```python
from build123d import *

# Parameters (mm, degrees)
F0_R     = 5.25
F0_R_2   = 4.25
F1_DEPTH = 6


with BuildPart() as f1:
    # F0 (on Front) → F1 (new body)
    with BuildSketch(Plane.XZ):
        with BuildLine():
            Line((-25, 25), (-25, 0))
            ThreePointArc((-25, 0), (0, -25), (25, 0))
            Line((25, 0), (25, 110))
            ThreePointArc((25, 110), (16.706063, 126.216291), (-1.296809, 128.982892))
            Line((-1.296809, 128.982892), (-167.871012, 73.728615))
            ThreePointArc((-167.871012, 73.728615), (-184.680107, 46.013484), (-160, 25))
            Line((-160, 25), (-25, 25))
        make_face()
        with Locations((-160, 50)):
            Circle(F0_R, mode=Mode.SUBTRACT)
        Circle(F0_R_2, mode=Mode.SUBTRACT)
    extrude(amount=F1_DEPTH)


solid = f1.part
```
Work out the finished part from the listing and answer in its coordinate system (mm). A direction names the side the tool comes from. Give positions to 0.01 mm unless a question says otherwise; leave off trailing zeros. Loops run counter-clockwise (first coordinate to the right, second up) from the corner with the lowest first, then second, coordinate; pieces in that order, holes last. Notation, with made-up numbers: (55, 86.5) -> (69, 86.5) arc R21 ccw to (69, 113.5) -> close; hole circle Ø2 at (69.25, 56.25). An arc over 180 degrees is marked (long way). Use CSV: the item, a comma, the result in double quotes.
1. The part is cut by section D-D (z = 86). Write down the section's boundary in (x, y).
Found:
outline,"(-130.88, -6) -> (25, -6) -> (25, 0) -> (-130.88, 0) -> close"
2. Flat-ended cylindrical pins translate along their axes: pin 1 Ø1.5 at (x, y) = (-29, -0.5) entering from +Z; pin 2 Ø9.5 at (x, z) = (-160, 50) entering from +Y. Find the tip coordinate at first contact, or state that the pin passes through.
Found:
pin 1,"z = 120.04"
pin 2,"through"
3. The part is cut by section B-B (y = -1.7). Write down the section's boundary in (x, z).
Found:
outline,"(-167.87, 73.73) arc R25 ccw to (-160, 25) -> (-25, 25) -> (-25, 0) arc R25 ccw to (25, 0) -> (25, 110) arc R20 ccw to (-1.3, 128.98) -> close; hole circle Ø10.5 at (-160, 50); hole circle Ø8.5 at (0, 0)"
4. A tool of negligible diameter and unlimited length cuts with its end or side. For faces 1 (the cylindrical face through (2.285, -2.958, 3.584)), 2 (the flat face through (-93, -3, 25)), from which of +Z, -Z, +X, -X, +Y, -Y can it reach the whole face along a straight path? Write none if from no direction.
Found:
face 1,"+Y, -Y"
face 2,"-Z, -X, +Y, -Y"
5. The mould has two halves that part along Z. Classify faces 3 (the flat face through (-83.42, -2.96, 101.74)), 4 (the flat face through (-25, -3, 13)), 5 (the cylindrical face through (-155, -3, 51.6)): +Z half, -Z half, draft (parallel to the pull), parting line (faces both ways), or undercut.
Found:
face 3,"+Z half"
face 4,"draft"
face 5,"undercut"
6. The part is cut by section A-A (z = 50). Write down the section's boundary in (x, y).
Found:
outline,"(-185, -6) -> (-165.25, -6) -> (-165.25, 0) -> (-185, 0) -> close; (-154.75, -6) -> (25, -6) -> (25, 0) -> (-154.75, 0) -> close"
7. The part is cut by section C-C (x = -130). Write down the section's boundary in (y, z).
Found:
outline,"(-6, 25) -> (0, 25) -> (0, 86.29) -> (-6, 86.29) -> close"
8. Straight lines are drawn through the part: line 1 (X direction, y = -3.95, z = 18); line 2 (Z direction, x = 0, y = -3.05); line 3 (X direction, y = -3.45, z = -2.5). For each, find the intervals that lie inside material, in ascending order.
Found:
line 1,"-25 to 25"
line 2,"-25 to -4.25, 4.25 to 129.36"
line 3,"-24.87 to -3.44, 3.44 to 24.87"
